from build123d import *

# Parameters (mm, degrees)
SKIZZE1_R                       = 19
AUFSATZ_LINEAR_AUSTRAGEN1_DEPTH = 4
M10_GEWINDEBOHRUNG1_D           = 8.5


with BuildPart() as part:
    # Skizze1 → Aufsatz-Linear austragen1 (new, symmetric)
    with BuildSketch(Plane.XY):
        with BuildLine():
            Line((0, 42.5), (10, 42.5))
            ThreePointArc((10, 42.5), (59.497474683, 63.002525317), (80, 112.5))
            Line((80, 112.5), (80, 117.5))
            Line((80, 117.5), (120, 157.5))
            Line((120, 157.5), (162.5, 157.5))
            Line((162.5, 157.5), (162.5, -42.5))
            Line((162.5, -42.5), (0, -42.5))
            ThreePointArc((0, -42.5), (-42.5, 0), (0, 42.5))
        make_face()
        Circle(SKIZZE1_R, mode=Mode.SUBTRACT)
    extrude(amount=AUFSATZ_LINEAR_AUSTRAGEN1_DEPTH, both=True)

    # M10 Gewindebohrung1 (through all)
    with Locations(Plane.XY.offset(4)):
        with Locations((25, -25), (25, 25)):
            Hole(M10_GEWINDEBOHRUNG1_D / 2)


solid = part.part
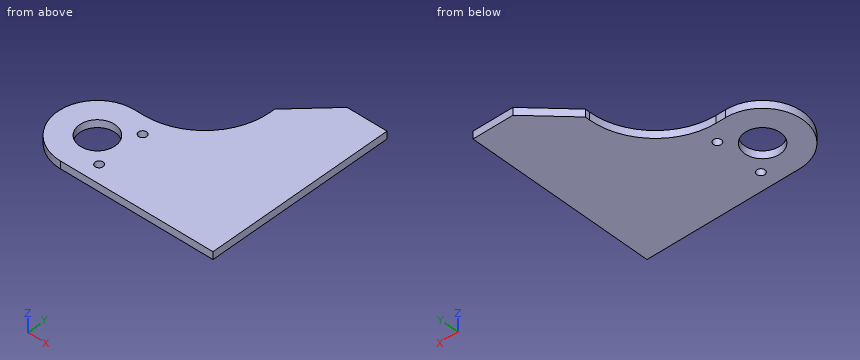
Read the model definition and answer for the solid it produces. Units are mm, in the model's axes. Coordinates: 2 decimals unless noted, no trailing zeros. Write each loop counter-clockwise with the first axis right and the second up, starting at its lowest first coordinate (ties: lowest second). Pieces come first, ordered by that corner, then holes. Notation, with made-up numbers: (-23.75, -39.75) - (-15.75, -39.75) arc R34 ccw to (-15.75, -6.75) - close; hole circle Ø10 at (84.5, 87). An arc over 180 degrees is marked (long way). One line per question, with ' | ' between items.
Q1. Find section A-A, the plane y = 0. Write down the section's boundary in (x, z), plus the area to 3 significant figures.
Result set:
outline: (-42.5, -4) - (-19, -4) - (-19, 4) - (-42.5, 4) - close; (19, -4) - (162.5, -4) - (162.5, 4) - (19, 4) - close | area: 1,340 mm^2
Q2. Consider L1, parallel to Y at x = 25, z = 0.75; L2, parallel to X at y = 22, z = 0; L3, parallel to Y at x = -17, z = 0. Determine where each line is inside the solid, lowest interval first. Write a range as [from, to].
Result set:
L1: [-42.5, -29.25], [-20.75, 20.75], [29.25, 44.13] | L2: [-36.36, 21.99], [28.01, 162.5] | L3: [-38.95, -8.49], [8.49, 38.95]
Q3. Each of these flat-tipped pins is pushed along its axis until it touches: P1, Ø3, axis at x = 22.5, z = -2, coming from the +Y side; P2, Ø5, axis at x = 25, y = -25, coming from the -Z side. Where does it stop, or does it pass through?
Result set:
P1: y = 43.91 | P2: through
Q4. Find section C-C, the plane x = 4.5. Write down the section's boundary in (y, z), plus the area to 3 significant figures.
Result set:
outline: (-42.5, -4) - (-18.46, -4) - (-18.46, 4) - (-42.5, 4) - close; (18.46, -4) - (42.5, -4) - (42.5, 4) - (18.46, 4) - close | area: 385 mm^2
Q5. Find section B-B, the plane z = -2. Write down the section's boundary in (x, y).
Result set:
outline: (0, -42.5) - (162.5, -42.5) - (162.5, 157.5) - (120, 157.5) - (80, 117.5) - (80, 112.5) arc R70 cw to (10, 42.5) - (0, 42.5) arc R42.5 ccw to start; hole circle Ø38 at (0, 0); hole circle Ø8.5 at (25, -25); hole circle Ø8.5 at (25, 25)
Q6. Find section D-D, the plane x = 25. Write down the section's boundary in (y, z).
Result set:
outline: (-42.5, -4) - (-29.25, -4) - (-29.25, 4) - (-42.5, 4) - close; (-20.75, -4) - (20.75, -4) - (20.75, 4) - (-20.75, 4) - close; (29.25, -4) - (44.13, -4) - (44.13, 4) - (29.25, 4) - close
